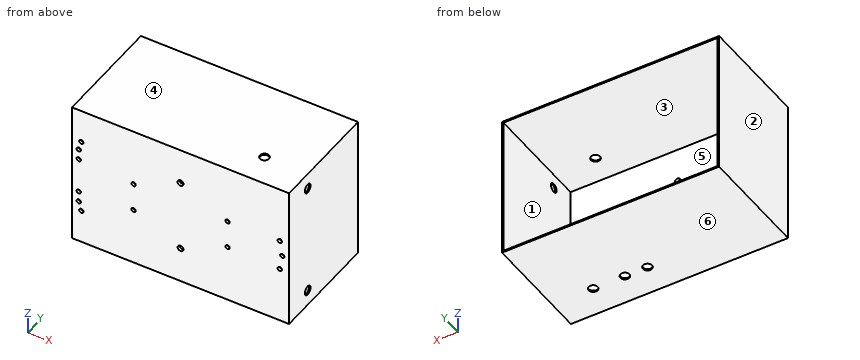
Autodesk Inventor part; units mm, degrees
ref_plane "YZ Plane" through (0, 0, 0) normal (1, 0, 0) x (0, 1, 0)
ref_plane "XZ Plane" through (0, 0, 0) normal (0, 1, 0) x (-1, 0, 0)
ref_plane "XY Plane" through (0, 0, 0) normal (0, 0, 1) x (1, 0, 0)
sketch "Sketch1" plane through (0, 0, 0) normal (0, 1, 0) x (-1, 0, 0)
  line L0 (-76.2, 50.8) -> (76.2, 50.8)
  line L1 (76.2, 50.8) -> (76.2, -50.8)
  line L2 (76.2, -50.8) -> (-76.2, -50.8)
  line L3 (-76.2, -50.8) -> (-76.2, 50.8)
  line L4 (-76.2, 50.8) -> (76.2, -50.8) construction
  line L5 (76.2, 50.8) -> (-76.2, -50.8) construction
  point P0 (0, 0)
  dimension "d0" = 152.4
  dimension "d1" = 101.6
extrude "Extrusion1" add sketch "Sketch1" along normal blind 2.032
sketch "Sketch2" plane through (0, 2.032, 0) normal (0, 1, 0) x (1, 0, 0)
  line L0 (-76.2, -50.8) -> (76.2, -50.8)
  line L1 (76.2, -50.8) -> (76.2, 50.8)
  line L2 (-76.2, -50.8) -> (76.2, -50.8)
  line L3 (76.2, -50.8) -> (76.2, 50.8)
  line L4 (76.2, 50.8) -> (-76.2, 50.8)
  line L5 (-76.2, 50.8) -> (-76.2, -50.8)
  line L6 (75.184, -49.784) -> (-75.184, -49.784)
  line L7 (-75.184, -49.784) -> (-75.184, 49.784)
  line L8 (-75.184, 49.784) -> (75.184, 49.784)
  line L9 (75.184, 49.784) -> (75.184, -49.784)
  line L10 (75.184, -49.784) -> (-75.184, 49.784) construction
  line L11 (-75.184, -49.784) -> (75.184, 49.784) construction
  point P0 (0, 0)
  dimension "d4" = 150.368
  dimension "d5" = 99.568
extrude "Extrusion2" add sketch "Sketch2" along normal blind 76.2
sketch "Sketch3" plane through (0, 2.032, 0) normal (0, 1, 0) x (1, 0, 0)
  circle A0 centre (0, -25.4) radius 2.0828
  circle A1 centre (0, 25.4) radius 2.0828
  point P0 (0, 0)
  dimension "d10" = 4.1656
  dimension "d11" = 4.1656
extrude "Extrusion3" cut sketch "Sketch3" against normal through all
sketch "Sketch4" plane through (0, 2.032, 0) normal (0, 1, 0) x (1, 0, 0)
  line L0 (32.9946, -9.9949) -> (-32.9946, 9.9949) construction
  line L1 (-32.9946, -9.9949) -> (32.9946, 9.9949) construction
  circle A0 centre (-32.9946, -9.9949) radius 1.4986
  circle A1 centre (-32.9946, 9.9949) radius 1.4986
  circle A2 centre (32.9946, 9.9949) radius 1.4986
  circle A3 centre (32.9946, -9.9949) radius 1.4986
  line L2 (-70.0024, -27.7812) -> (70.0024, 27.7812) construction
  line L3 (70.0024, -27.7812) -> (-70.0024, 27.7812) construction
  line L4 (70.6437, -27.7812) -> (-70.6437, 27.7812) construction
  line L5 (-70.6437, -27.7812) -> (70.6437, 27.7812) construction
  line L6 (70.6437, -27.7812) -> (86.5188, -27.7812) construction
  circle A4 centre (-71.4565, 20.1613) radius 1.524
  circle A5 centre (-71.4565, 12.5413) radius 1.524
  circle A6 centre (-71.4565, -12.5413) radius 1.524
  circle A7 centre (-71.4565, -20.1613) radius 1.524
  circle A8 centre (-69.6277, -26.7653) radius 1.524
  circle A9 centre (-69.6277, 26.7653) radius 1.524
  circle A10 centre (69.6277, -10.8903) radius 1.524
  circle A11 centre (71.4565, 0) radius 1.524
  circle A12 centre (69.6277, 10.8903) radius 1.524
  point P0 (0, 0)
  point P1 (0, 0)
  dimension "d14" = 65.9892
  dimension "d15" = 19.9898
  dimension "d16" = 2.9972
  dimension "d17" = 2.9972
  dimension "d18" = 2.9972
  dimension "d19" = 2.9972
  dimension "d21" = 55.5625
  dimension "d62" = 141.2875
  dimension "d63" = 55.5625
  dimension "d96" = 3.048
  dimension "d97" = 3.048
  dimension "d98" = 3.048
  dimension "d99" = 3.048
  dimension "d103" = 3.048
  dimension "d106" = 3.048
  dimension "d111" = 3.048
  dimension "d112" = 3.048
  dimension "d113" = 3.048
sketch "Sketch5" plane through (-75.184, 2.032, -49.784) normal (0, 0, 1) x (1, 0, 0)
  line L0 (151.384, 76.2) -> (-1.016, 76.2)
  line L1 (0.0002, 76.2) -> (150.368, 76.2)
  line L2 (150.368, 76.2) -> (150.368, 0)
  line L3 (150.368, 0) -> (0.0002, 0)
  line L4 (0.0002, 0) -> (0.0002, 76.2)
  circle A0 centre (84.5566, 19.05) radius 3.175
  circle A1 centre (100.4316, 19.05) radius 3.175
  circle A2 centre (122.6566, 19.05) radius 3.175
  point P0 (75.184, -2.032)
  dimension "d39" = 6.35
  dimension "d40" = 6.35
  dimension "d41" = 6.35
extrude "Extrusion5" cut sketch "Sketch5" against normal through all contours A0 | A1 | A2
sketch "Sketch6" plane through (75.184, 2.032, -49.784) normal (-1, 0, 0) x (0, 0, 1)
  circle A0 centre (10.16, 19.05) radius 3.175
  circle A1 centre (89.408, 19.05) radius 3.175
  point P0 (49.784, -2.032)
  dimension "d44" = 6.35
  dimension "d45" = 6.35
extrude "Extrusion6" cut sketch "Sketch6" against normal through all
sketch "Sketch7" plane through (75.184, 2.032, 49.784) normal (0, 0, -1) x (-1, 0, 0)
  line L0 (150.368, 0) -> (150.368, 76.2)
  line L1 (150.368, 19.05) -> (155.5496, 19.05) construction
  circle A0 centre (29.2989, 19.05) radius 3.175
  point P0 (75.184, -2.032)
  dimension "d51" = 6.35
extrude "Extrusion7" cut sketch "Sketch7" against normal through all
extrude "Extrusion8" cut sketch "Sketch4" against normal through all
properties part number "546-1444-8-ADF4355"
For this review, take the finished solid that the model builds, in its own axes (mm). Face numbers are marked on the shaded views. A direction names the side the tool comes from. Round coordinates to 2 decimals unless told otherwise and drop trailing zeros. Write each loop counter-clockwise with the first axis right and the second up, starting at its lowest first coordinate (ties: lowest second). Pieces come first, ordered by that corner, then holes. Notation, with made-up numbers: (63, 9.5) -> (72, 9.5) arc R20 ccw to (72, 42.5) -> close; hole circle Ø9 at (-29, 78.25). An arc over 180 degrees is marked (long way). Use one line per item in the form item = value.
Q1. Consider section C-C (z = -4.5). State the section outline as (x, y) points, then the cut area to 3 significant figures.
Resolved:
outline = (-76.2, 0) -> (76.2, 0) -> (76.2, 78.23) -> (75.18, 78.23) -> (75.18, 2.03) -> (-75.18, 2.03) -> (-75.18, 78.23) -> (-76.2, 78.23) -> close
area = 465 mm²
Q2. Clearance check with flat-ended pins moving along their axes: pin 1 Ø2.5 at (x, z) = (-71.46, 12.54) entering from +Y; pin 2 Ø5 at (y, z) = (21.082, 39.624) entering from +X; pin 3 Ø5 at (x, z) = (23.5, -2.5) entering from +Y. State where each tip first meets the part, or that it passes through.
Resolved:
pin_1 = through
pin_2 = -75.18
pin_3 = 2.03
Q3. Consider section B-B (y = 11). State the section outline as (x, z) points, then the cut area to 3 significant figures.
Resolved:
outline = (-76.2, -50.8) -> (76.2, -50.8) -> (76.2, 50.8) -> (-76.2, 50.8) -> close; hole (-75.18, -49.78) -> (75.18, -49.78) -> (75.18, 49.78) -> (-75.18, 49.78) -> close
area = 512 mm²
Q4. The part is to be moulded in two halves that separate along X. For the marked faces 1, 2, 3 and 4, say which applies: released by +X, released by -X, zero draft, split by the parting line, or undercut.
Resolved:
face_1 = undercut
face_2 = released by -X
face_3 = undercut
face_4 = zero draft
Q5. Machinability: for the marked faces 5 and 6, which of the approach directions +Z, -Z, +X, -X, +Y, -Y give a long, thin tool a straight path to every point of the face, cutting with its end or side? Answer none if there is none.
Resolved:
face_5 = +Y
face_6 = -Z, +X, -X, +Y, -Y
Q6. Consider section A-A (x = 0). State the section outline as (y, z) points.
Resolved:
outline = (0, -50.8) -> (78.23, -50.8) -> (78.23, -49.78) -> (2.03, -49.78) -> (2.03, -27.48) -> (0, -27.48) -> close; (0, -23.32) -> (2.03, -23.32) -> (2.03, 23.32) -> (0, 23.32) -> close; (0, 27.48) -> (2.03, 27.48) -> (2.03, 49.78) -> (78.23, 49.78) -> (78.23, 50.8) -> (0, 50.8) -> close
Q7. To check wall thickness, follow probe 1 along X at (y, z) = (47, 32); probe 2 along X at (y, z) = (1.05, 0); probe 3 along Z at (x, y) = (55, 28.5). State the ranges of each line that lie inside material, in increasing order. Write a range as from..to.
Resolved:
probe_1 = -76.2..-75.18, 75.18..76.2
probe_2 = -76.2..69.93, 72.98..76.2
probe_3 = -50.8..-49.78, 49.78..50.8
Q8. Consider section D-D (x = -65.5). State the section outline as (y, z) points.
Resolved:
outline = (0, -50.8) -> (78.23, -50.8) -> (78.23, -49.78) -> (2.03, -49.78) -> (2.03, 49.78) -> (78.23, 49.78) -> (78.23, 50.8) -> (0, 50.8) -> close
